from build123d import *

# Parameters (mm, degrees)
BOSS_EXTRUDE1_DEPTH = 6.35
FILLET1_R           = 2.54
SKETCH2_R           = 2.54
CUT_EXTRUDE1_DEPTH  = 6.35


with BuildPart() as part:
    # Sketch1 → Boss-Extrude1 (new body)
    with BuildSketch(Plane(origin=(0, 0, 0), x_dir=(1, 0, 0), z_dir=(0, 1, 0))):
        Polygon((0, -49.53), (0, 49.53), (-18.074412074, 71.12), (-33.314412074, 71.12), (-15.24, 49.53), (-15.24, -49.53), (-33.314412074, -71.12), (-18.074412074, -71.12), align=None)
    extrude(amount=BOSS_EXTRUDE1_DEPTH)

    # Fillet1
    fillet1_edges = [part.edges().sort_by_distance(p)[0] for p in [
        (-15.24, 0, 0),
        (-24.277206037, 0, -60.325),
        (-25.694412074, 0, -71.12),
        (-9.037206037, 0, -60.325),
        (-24.277206037, 6.35, -60.325),
        (0, 3.175, -49.53),
        (0, 3.175, 49.53),
        (-18.074412074, 3.175, 71.12),
        (-33.314412074, 3.175, 71.12),
        (-15.24, 3.175, 49.53),
        (-15.24, 3.175, -49.53),
        (-33.314412074, 3.175, -71.12),
        (-18.074412074, 3.175, -71.12),
        (-15.24, 6.35, 0),
        (-24.277206037, 6.35, 60.325),
        (-25.694412074, 6.35, 71.12),
        (-9.037206037, 6.35, 60.325),
        (0, 6.35, 0),
        (-9.037206037, 6.35, -60.325),
        (0, 0, 0),
        (-25.694412074, 6.35, -71.12),
        (-9.037206037, 0, 60.325),
        (-25.694412074, 0, 71.12),
        (-24.277206037, 0, 60.325),
    ]]
    fillet(fillet1_edges, radius=FILLET1_R)

    # Sketch2 → Cut-Extrude1 (cut)
    with BuildSketch(Plane(origin=(0, 6.35, 0), x_dir=(1, 0, 0), z_dir=(0, 1, 0))):
        with Locations((-21.19842308, -65.532)):
            Circle(SKETCH2_R)
    cut_extrude1 = extrude(amount=-CUT_EXTRUDE1_DEPTH, mode=Mode.SUBTRACT)

    # Mirror1: Cut-Extrude1 across plane
    add(cut_extrude1.mirror(Plane.XY), mode=Mode.SUBTRACT)


solid = part.part
Here's how the part is built. I have some questions about the finished solid (model axes, mm). A direction names the side the tool comes from. Coordinates: 2 decimals unless noted, no trailing zeros. Write each loop counter-clockwise with the first axis right and the second up, starting at its lowest first coordinate (ties: lowest second). Pieces come first, ordered by that corner, then holes.
Item 1: If we mould it in two halves opening along X, with no side actions, what happens to faces 6 (the cylindrical face through (-23.21, 3.22, 67.08)), 7 (the flat face through (-10, 6.35, -1)), 8 (the flat face through (-22.926, 3.166, -58.711))? For each: +X half, -X half, draft (parallel to the pull), parting line (faces both ways), or undercut.
Item 2: Will these pins go through, and if not, where does the flat tip stop? pin 1 (3 mm diameter, centred on y = 5.5, z = -31, fed in from +X); pin 2 (1 mm diameter, centred on y = 3, z = -2, fed in from -X).
Item 3: I want a section at A-A on z = -33. Write out the boundary of the cut face in (x, y), and give its area (3 significant figures).
Item 4: On a 3-axis mill with a long thin cutter (end or side, diameter ignored), from which of +Z, -Z, +X, -X, +Y, -Y can I reach the whole of each face in a straight line? I mean faces 1 (the flat face through (-22.73, 3.166, 58.477)), 2 (the cylindrical face through (-14.516, 0.764, 0.681)), 3 (the cylindrical face through (-14.5, 5.6, 0.7)), 4 (the cylindrical face through (-0.724, 0.764, -0.681)), 5 (the cylindrical face through (-9.391, 0.764, 59.619)). Say none if no direction works.
Item 5: I want a section at B-B on y = 1.25. Write out the boundary of the cut face in (x, z), and give its area (3 significant figures).
Item 6: If I drill on line 1 (Z direction, x = -21, y = 2.25); line 2 (Z direction, x = -22.5, y = 3.75); line 3 (X direction, y = 2.25, z = -48.5), over which ranges is the centre line in solid material (lowest first)?
Item 7: I want a section at C-C on x = -20.5. Count the separate pieces of the cut face and the enclosed holes in it, and give its area (3 significant figures).
Findings below:
1. face 6: undercut
1. face 7: draft
1. face 8: -X half
2. pin 1: stops at x = -0.01
2. pin 2: stops at x = -15.24
3. outline: (-15.24, 2.54) arc R2.54 ccw to (-12.7, 0) - (-2.54, 0) arc R2.54 ccw to (0, 2.54) - (0, 3.81) arc R2.54 ccw to (-2.54, 6.35) - (-12.7, 6.35) arc R2.54 ccw to (-15.24, 3.81) - close
3. area: 91.2 mm2
4. face 1: -X, +Y, -Y
4. face 2: -X, -Y
4. face 3: -X, +Y
4. face 4: +Z, -Z, +X, -Y
4. face 5: +Z, +X, -Y
5. outline: (-29.55, -67.18) arc R2.19 ccw to (-27.88, -70.77) - (-19.26, -70.77) arc R2.19 ccw to (-17.58, -69.98) - (-0.86, -50.01) arc R2.19 ccw to (-0.35, -48.61) - (-0.35, 48.61) arc R2.19 ccw to (-0.86, 50.01) - (-17.58, 69.98) arc R2.19 ccw to (-19.26, 70.77) - (-27.88, 70.77) arc R2.19 ccw to (-29.55, 67.18) - (-15.56, 50.46) arc R2.89 cw to (-14.89, 48.61) - (-14.89, -48.61) arc R2.89 cw to (-15.56, -50.46) - close; hole circle Ø5.08 at (-21.2, -65.53); hole circle Ø5.08 at (-21.2, 65.53)
5. area: 2,000 mm2
6. line 1: z = -71.1 to -68.06, -63 to -56.44, 56.44 to 63, 68.06 to 71.1
6. line 2: z = -71.12 to -67.71, -63.35 to -58.2, 58.2 to 63.35, 67.71 to 71.12
6. line 3: x = -15.22 to -0.02
7. separate pieces: 4
7. enclosed holes: 0
7. area: 118 mm2
